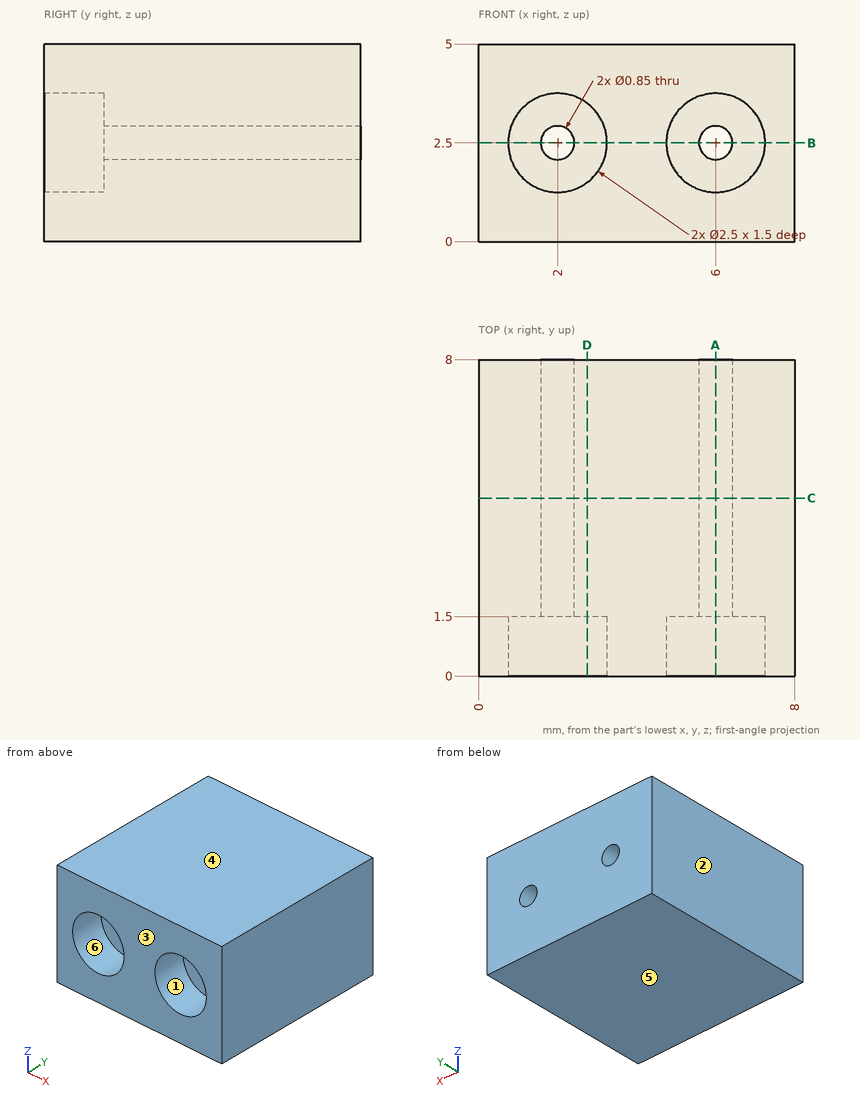
Input: dimensioned drawing with shaded views. Units: mm. Origin: part minimum x, y, z. A direction names the side the tool comes from. Round coordinates to 2 decimals unless told otherwise and drop trailing zeros. Write each loop counter-clockwise with the first axis right and the second up, starting at its lowest first coordinate (ties: lowest second). Pieces come first, ordered by that corner, then holes. Notation, with made-up numbers: (-10.75, 66) - (23.25, 66) arc R25 ccw to (23.25, 91) - close; hole circle Ø5 at (13, 5.25). An arc over 180 degrees is marked (long way). Write item = value, one per line.
(1) Section query C-C on y = 4.5. Output: boundary loops of the cut face in (x, z) (3 decimals).
Geometry check:
outline = (0, 0) - (8, 0) - (8, 5) - (0, 5) - close; hole circle Ø0.85 at (2, 2.5); hole circle Ø0.85 at (6, 2.5)
(2) Material intervals for probe 1 along Z at (x, y) = (2, 6) (3 decimals); probe 2 along Z at (x, y) = (6, 0.7); probe 3 along X at (y, z) = (4.25, 2.3) (3 decimals), sorted ascending.
Geometry check:
probe_1 = 0 to 2.075, 2.925 to 5
probe_2 = 0 to 1.25, 3.75 to 5
probe_3 = 0 to 1.625, 2.375 to 5.625, 6.375 to 8
(3) Access query for the marked faces 1 and 2. Directions: +Z, -Z, +X, -X, +Y, -Y. A direction counts if a zero-diameter tool reaches every point of the face in a straight line with its end or side. Return the directions, or none.
Geometry check:
face_1 = -Y
face_2 = +Z, -Z, -X, +Y, -Y
(4) Pull-direction query (Z, two-part tool) for the marked faces 3, 4, 5 and 6; classes: +Z half, -Z half, draft (parallel to the pull), parting line (faces both ways), or undercut.
Geometry check:
face_3 = draft
face_4 = +Z half
face_5 = -Z half
face_6 = undercut
(5) Section query A-A on x = 6. Output: boundary loops of the cut face in (y, z) (3 decimals), then the cut area to 3 significant figures.
Geometry check:
outline = (0, 0) - (8, 0) - (8, 2.075) - (1.5, 2.075) - (1.5, 1.25) - (0, 1.25) - close; (0, 3.75) - (1.5, 3.75) - (1.5, 2.925) - (8, 2.925) - (8, 5) - (0, 5) - close
area = 30.7 mm^2
(6) Contact query for a flat-ended pin moving along its axis: pin 1 Ø1.2 at (x, z) = (6, 2) entering from -Y. Output: stop coordinate, or through.
Geometry check:
pin_1 = 1.5
(7) Section query D-D on x = 2.75. Output: boundary loops of the cut face in (y, z), then the cut area to 3 significant figures.
Geometry check:
outline = (0, 0) - (8, 0) - (8, 5) - (0, 5) - (0, 3.5) - (1.5, 3.5) - (1.5, 1.5) - (0, 1.5) - close
area = 37.0 mm^2
(8) Section query B-B on z = 2.5. Output: boundary loops of the cut face in (x, y) (3 decimals), then the cut area to 4 significant figures.
Geometry check:
outline = (0, 0) - (0.75, 0) - (0.75, 1.5) - (1.575, 1.5) - (1.575, 8) - (0, 8) - close; (2.425, 1.5) - (3.25, 1.5) - (3.25, 0) - (4.75, 0) - (4.75, 1.5) - (5.575, 1.5) - (5.575, 8) - (2.425, 8) - close; (6.425, 1.5) - (7.25, 1.5) - (7.25, 0) - (8, 0) - (8, 8) - (6.425, 8) - close
area = 45.45 mm^2
